```python
from build123d import *

# Parameters (mm, degrees)
SKETCH1_R           = 4.93
BOSS_EXTRUDE1_DEPTH = 6.06
SKETCH2_R           = 3
BOSS_EXTRUDE2_DEPTH = 30
SKETCH3_R           = 5.935
BOSS_EXTRUDE3_DEPTH = 1.02


with BuildPart() as part:
    # Sketch1 → Boss-Extrude1 (new body)
    with BuildSketch(Plane(origin=(0, 0, 0), x_dir=(0, 0, -1), z_dir=(1, 0, 0))):
        Circle(SKETCH1_R)
    extrude(amount=BOSS_EXTRUDE1_DEPTH)

    # Sketch2 → Boss-Extrude2 (add)
    with BuildSketch(Plane.ZY):
        Circle(SKETCH2_R)
    extrude(amount=BOSS_EXTRUDE2_DEPTH)

    # Sketch3 → Boss-Extrude3 (add)
    with BuildSketch(Plane.ZY):
        Circle(SKETCH3_R)
    extrude(amount=BOSS_EXTRUDE3_DEPTH)


solid = part.part
```
Verification items for the finished model (mm, model axes). A direction names the side the tool comes from. Round coordinates to 2 decimals unless told otherwise and drop trailing zeros. Order: outer loops, then holes, each group sorted by start corner. A loop starts at its lowest first (then second) coordinate and runs counter-clockwise, first axis right, second up.
1) Tool access check on faces 1 (the flat face through (-1.02, 1, -3)), 2 (the flat face through (-30, 0, 0)), 3 (the flat face through (0, 5, 1)). Record the directions out of +Z, -Z, +X, -X, +Y, -Y that give a thin tool (end or side, any length) a straight path to the whole face; none if there is none.
Geometry says:
face 1: -X
face 2: +Z, -Z, -X, +Y, -Y
face 3: +X
2) Cross-section at A-A, the plane y = 0. Record the cut outline in (x, z) (3 decimals).
Geometry says:
outline: (-30, -3) - (-1.02, -3) - (-1.02, -5.935) - (0, -5.935) - (0, -4.93) - (6.06, -4.93) - (6.06, 4.93) - (0, 4.93) - (0, 5.935) - (-1.02, 5.935) - (-1.02, 3) - (-30, 3) - close
3) Material ranges on line 1 (X direction, y = -1, z = -3.5); line 2 (Y direction, x = 3, z = 4); line 3 (Y direction, x = -3, z = -2.25), recorded low to high.
Geometry says:
line 1: x = -1.02 to 6.06
line 2: y = -2.88 to 2.88
line 3: y = -1.98 to 1.98
4) Depth check by flat-ended pin: pin 1 (6 mm diameter, centred on x = -7, z = -4, fed in from +Y); pin 2 (6 mm diameter, centred on x = -13.5, z = 2, fed in from -Y); pin 3 (1.5 mm diameter, centred on x = -9.5, z = -3.5, fed in from +Y). Enter the tip coordinate at first touch or a pass-through.
Geometry says:
pin 1: stops at y = 2.83
pin 2: stops at y = -3
pin 3: stops at y = 1.2
5) Cross-section at D-D, the plane y = -4. Record the cut outline in (x, z).
Geometry says:
outline: (-1.02, -4.38) - (0, -4.38) - (0, -2.88) - (6.06, -2.88) - (6.06, 2.88) - (0, 2.88) - (0, 4.38) - (-1.02, 4.38) - close
6) Cross-section at C-C, the plane x = -22. Record the cut outline in (y, z), plus the area to 3 significant figures.
Geometry says:
outline: circle Ø6 at (0, 0)
area: 28.3 mm2
